Autodesk Inventor part; units mm, degrees
ref_plane "YZ Plane" through (0, 0, 0) normal (1, 0, 0) x (0, 1, 0)
ref_plane "XZ Plane" through (0, 0, 0) normal (0, 1, 0) x (-1, 0, 0)
ref_plane "XY Plane" through (0, 0, 0) normal (0, 0, 1) x (1, 0, 0)
ref_plane "Work Plane1" through (22.5184, 2.463, -18.3509) normal (0, 0, 1) x (0.9997722, -0.0213418, 0)
sketch "ThermoBulbBorder" plane through (22.5184, 2.463, -18.3509) normal (0, 0, 1) x (0.9997722, -0.0213418, 0)
  arc A0 (-447.455, -468.958) -> (162.145, -468.958) centre (-142.655, -774.8145) ccw
  arc A1 (-447.455, -468.958) -> (162.145, -468.958) centre (-142.655, -774.8145) ccw
  arc A2 (-383.955, -588.5959) -> (98.645, -588.5959) centre (-142.655, -774.8145) ccw
  line L0 (-447.455, -468.958) -> (-383.955, -468.958)
  line L1 (-383.955, -468.958) -> (-383.955, -588.5959)
  line L2 (162.145, -468.958) -> (98.645, -468.958)
  line L3 (98.645, -468.958) -> (98.645, -588.5959)
  line L4 (-383.955, -961.033) -> (-484.4967, -1038.6241)
  line L5 (98.645, -961.033) -> (199.1867, -1038.6241)
  arc A3 (-447.455, -468.958) -> (162.145, -468.958) centre (-142.655, -774.8145) ccw
  circle A4 centre (-142.655, -774.8145) radius 419.1 construction
  circle A5 centre (-142.655, -774.8145) radius 410.972 construction
  circle A6 centre (-142.655, -774.8145) radius 353.822 construction
  circle A7 centre (-142.655, -774.8145) radius 345.694 construction
  line L6 (98.645, -468.958) -> (98.645, -316.558) construction
  line L7 (-383.955, -468.958) -> (-383.955, -316.558) construction
  dimension "d0" = 609.6
  dimension "d5" = 63.5
  dimension "d6" = 63.5
  dimension "d7" = 838.2
  dimension "d8" = 8.128
  dimension "d9" = 8.128
  dimension "d10" = 57.15
  dimension "d11" = 40.894
  dimension "d12" = 152.4
extrude "Sides" add sketch "ThermoBulbBorder" along normal blind 18.034 contours L0 L1 A2 L4 A0 | L5 A2 L3 L2 A0
extrude "Extrusion2" add sketch "ThermoBulbBorder" along normal blind 18.034 contours L4 A2 L5 A0
equation "\"d6\" = d5"
equation "\"d8\" = sRopeChannel"
equation "\"d9\" = sRopeChannel"
equation "\"sRopeChannel\" = 8.128"
properties part number "HOT Thermo bulb outline"
Could you check a few things on this model? Use its own coordinates, in mm. Round coordinates to 2 decimals unless told otherwise and drop trailing zeros. Write each loop counter-clockwise with the first axis right and the second up, starting at its lowest first coordinate (ties: lowest second). Pieces come first, ordered by that corner, then holes. Notation, with made-up numbers: (86.5, 49.25) -> (140.5, 49.25) arc R20 ccw to (140.5, 80.25) -> close; hole circle Ø4 at (-2.75, 32.25). An arc over 180 degrees is marked (long way). Use a Markdown table: item, result.
1. If we section it at B-B (y = -887): List the corners of the cut face in (x, z) for me.
Answer key:
| item | result |
|---|---|
| outline | (-552.04, -18.35) -> (-417.73, -18.35) -> (-417.73, -0.32) -> (-552.04, -0.32) -> close; (144.45, -18.35) -> (278.76, -18.35) -> (278.76, -0.32) -> (144.45, -0.32) -> close |
2. For pin 1 Ø5 at (x, z) = (-239, -13) entering from -Y; pin 2 Ø8 at (x, z) = (-343.5, -15) entering from -Y; pin 3 Ø4 at (y, z) = (-834.5, -10) entering from +X, each with a flat end and sliding along its axis, tell me the tip position at first contact or that it passes through.
Answer key:
| item | result |
|---|---|
| pin 1 | stops at y = -1189.22 |
| pin 2 | stops at y = -1150.31 |
| pin 3 | stops at x = 290.48 |
3. If we section it at C-C (z = -10.25): List the corners of the cut face in (x, y) for me.
Answer key:
| item | result |
|---|---|
| outline | (-434.84, -456.84) arc R431.8 ccw (long way) to (174.62, -469.85) -> (111.13, -468.49) -> (108.58, -588.1) arc R304.8 cw (long way) to (-373.91, -577.8) -> (-371.36, -458.19) -> close |
4. If we section it at D-D (x = -317): List the corners of the cut face in (y, z) for me.
Answer key:
| item | result |
|---|---|
| outline | (-1161.46, -18.35) -> (-1014.84, -18.35) -> (-1014.84, -0.32) -> (-1161.46, -0.32) -> close |
5. Please list where these lines run through material, in increasing order: probe 1 along Y at (x, z) = (-126.5, -5); probe 2 along X at (y, z) = (-791, -13); probe 3 along X at (y, z) = (-817.5, -2.5).
Answer key:
| item | result |
|---|---|
| probe 1 | y = -1200.81 to -1073.76 |
| probe 2 | x = -567.89 to -440.65, 167.37 to 294.61 |
| probe 3 | x = -565.72 to -437.58, 164.3 to 292.44 |
6. If we section it at A-A (x = 146): List the corners of the cut face in (y, z) for me, then the cut area to 3 significant figures.
Answer key:
| item | result |
|---|---|
| outline | (-1095.57, -18.35) -> (-883.23, -18.35) -> (-883.23, -0.32) -> (-1095.57, -0.32) -> close; (-655.04, -18.35) -> (-469.24, -18.35) -> (-469.24, -0.32) -> (-655.04, -0.32) -> close |
| area | 7,180 mm^2 |
7. We'd pull the mould along X, two halves only. Please class faces 1 (the face through (-133.638, -1073.916, -9.46)), 2 (the face through (-145, -1076, -0.317)), 3 (the face through (-131.6, -1200.9, -9.5)): +X half, -X half, draft (parallel to the pull), parting line (faces both ways), or undercut.
Answer key:
| item | result |
|---|---|
| face 1 | undercut |
| face 2 | draft |
| face 3 | parting line |
